Here's how the part is built. I have some questions about the finished solid (model axes, mm). A direction names the side the tool comes from. Coordinates: 2 decimals unless noted, no trailing zeros. Loops run counter-clockwise (first coordinate to the right, second up) from the corner with the lowest first, then second, coordinate; pieces in that order, holes last. Notation, with made-up numbers: (44.5, 52) -> (51.5, 52) arc R24 ccw to (51.5, 78) -> close; hole circle Ø2 at (82.25, -36). An arc over 180 degrees is marked (long way). Use CSV: the item, a comma, the result in double quotes. Start each with the question number.
from build123d import *

# Parameters (mm, degrees)
EXTRUDE_1_DEPTH = 2.2


with BuildPart() as part:
    # Model → 凸台-拉伸1 (new body)
    with BuildSketch(Plane.XY):
        Polygon((-11.407474747, -25.191111111), (-11.407474747, -22.191111111), (-16.407474747, -22.191111111), (-16.407474747, -19.191111111), (-21.407474747, -19.191111111), (-21.407474747, -14.191111111), (-23.407474747, -14.191111111), (-23.407474747, -4.191111111), (-21.407474747, -4.191111111), (-21.407474747, 5.808888889), (-23.407474747, 5.808888889), (-23.407474747, 15.808888889), (-21.407474747, 15.808888889), (-21.407474747, 20.808888889), (-16.407474747, 20.808888889), (-16.407474747, 23.808888889), (-11.407474747, 23.808888889), (-11.407474747, 26.808888889), (-1.407474747, 26.808888889), (-1.407474747, 23.808888889), (3.592525253, 23.808888889), (3.592525253, 26.808888889), (13.592525253, 26.808888889), (13.592525253, 23.808888889), (18.592525253, 23.808888889), (18.592525253, 20.808888889), (23.592525253, 20.808888889), (23.592525253, 15.808888889), (25.592525253, 15.808888889), (25.592525253, 5.808888889), (23.592525253, 5.808888889), (23.592525253, -4.191111111), (25.592525253, -4.191111111), (25.592525253, -14.191111111), (23.592525253, -14.191111111), (23.592525253, -19.191111111), (18.592525253, -19.191111111), (18.592525253, -22.191111111), (13.592525253, -22.191111111), (13.592525253, -25.191111111), (3.592525253, -25.191111111), (3.592525253, -22.191111111), (-1.407474747, -22.191111111), (-1.407474747, -25.191111111), align=None)
        with BuildLine():
            Line((16.092525253, 13.808888889), (15.092525253, 13.808888889))
            ThreePointArc((15.092525253, 13.808888889), (14.031865081, 14.248228717), (13.592525253, 15.308888889))
            Line((13.592525253, 15.308888889), (13.592525253, 16.308888889))
            ThreePointArc((13.592525253, 16.308888889), (13.153185424, 17.369549061), (12.092525253, 17.808888889))
            Line((12.092525253, 17.808888889), (-9.907474747, 17.808888889))
            ThreePointArc((-9.907474747, 17.808888889), (-10.968134919, 17.369549061), (-11.407474747, 16.308888889))
            Line((-11.407474747, 16.308888889), (-11.407474747, 15.308888889))
            ThreePointArc((-11.407474747, 15.308888889), (-11.846814576, 14.248228717), (-12.907474747, 13.808888889))
            Line((-12.907474747, 13.808888889), (-13.907474747, 13.808888889))
            ThreePointArc((-13.907474747, 13.808888889), (-14.968134919, 13.369549061), (-15.407474747, 12.308888889))
            Line((-15.407474747, 12.308888889), (-15.407474747, -10.691111111))
            ThreePointArc((-15.407474747, -10.691111111), (-14.968134919, -11.751771283), (-13.907474747, -12.191111111))
            Line((-13.907474747, -12.191111111), (-12.907474747, -12.191111111))
            ThreePointArc((-12.907474747, -12.191111111), (-11.846814576, -12.630450939), (-11.407474747, -13.691111111))
            Line((-11.407474747, -13.691111111), (-11.407474747, -14.691111111))
            ThreePointArc((-11.407474747, -14.691111111), (-10.968134919, -15.751771283), (-9.907474747, -16.191111111))
            Line((-9.907474747, -16.191111111), (12.092525253, -16.191111111))
            ThreePointArc((12.092525253, -16.191111111), (13.153185424, -15.751771283), (13.592525253, -14.691111111))
            Line((13.592525253, -14.691111111), (13.592525253, -13.691111111))
            ThreePointArc((13.592525253, -13.691111111), (14.031865081, -12.630450939), (15.092525253, -12.191111111))
            Line((15.092525253, -12.191111111), (16.092525253, -12.191111111))
            ThreePointArc((16.092525253, -12.191111111), (17.153185424, -11.751771283), (17.592525253, -10.691111111))
            Line((17.592525253, -10.691111111), (17.592525253, 12.308888889))
            ThreePointArc((17.592525253, 12.308888889), (17.153185424, 13.369549061), (16.092525253, 13.808888889))
        make_face(mode=Mode.SUBTRACT)
    extrude(amount=EXTRUDE_1_DEPTH)


solid = part.part
1) I want a section at B-B, the plane y = 14.5. Please give me the cut outline in (x, z).
2) I want a section at A-A, the plane x = -6.5. Please give me the cut outline in (y, z).
3) Please list where these lines run through material, in increasing order: L1, parallel to X at y = 11, z = 0.9; L2, parallel to Y at x = 2, z = 0.75; L3, parallel to X at y = 16.5, z = 0.6. Write a range as [from, to].
4) I want a section at D-D, the plane y = 22. Please give me the cut outline in (x, z), plus the area to 3 significant figures.
5) I want a section at C-C, the plane x = 20.5. Please give me the cut outline in (y, z), plus the area to 3 significant figures.
6) Thinking about a two-plate mould opening in X: for faces 1 (the face through (13.593, 25, 1)), 2 (the face through (-14.96, 13.38, 1.08)), 3 (the face through (16, -22.191, 1)), which applies, pulls with the +X half, pulls with the -X half, needs draft (parallel to the pull), parting line crosses it, or undercut?
7) For P1, Ø0.7, axis at y = 17.5, z = 1, coming from the -X side; P2, Ø0.7, axis at x = 0.5, z = 1, coming from the -Y side; P3, Ø0.6, axis at x = 24, z = 1, coming from the -Y side, each with a flat end and sliding along its axis, tell me the tip position at first contact or that it passes through.
8) Which directions (+Z, -Z, +X, -X, +Y, -Y) give clear straight access to the entire face, cutting with the end or side of a thin tool? Please do faces 4 (the face through (3.593, 25, 1)), 5 (the face through (-22, -4.191, 1)), 6 (the face through (17.1, -11.8, 1.1)), 7 (the face through (-11.407, 25, 1)), 8 (the face through (25, -14.191, 1)).
Return value:
1,outline,"(-23.41, 0) -> (-11.64, 0) -> (-11.64, 2.2) -> (-23.41, 2.2) -> close; (13.83, 0) -> (25.59, 0) -> (25.59, 2.2) -> (13.83, 2.2) -> close"
2,outline,"(-25.19, 0) -> (-16.19, 0) -> (-16.19, 2.2) -> (-25.19, 2.2) -> close; (17.81, 0) -> (26.81, 0) -> (26.81, 2.2) -> (17.81, 2.2) -> close"
3,L1,"x = [-23.41, -15.41], [17.59, 25.59]"
3,L2,"y = [-22.19, -16.19], [17.81, 23.81]"
3,L3,"x = [-21.41, -11.4], [13.58, 23.59]"
4,outline,"(-16.41, 0) -> (18.59, 0) -> (18.59, 2.2) -> (-16.41, 2.2) -> close"
4,area,"77.0 mm²"
5,outline,"(-19.19, 0) -> (20.81, 0) -> (20.81, 2.2) -> (-19.19, 2.2) -> close"
5,area,"88.0 mm²"
6,face 1,"pulls with the +X half"
6,face 2,"undercut"
6,face 3,"needs draft"
7,P1,"stops at x = -21.41"
7,P2,"stops at y = -22.19"
7,P3,"stops at y = -14.19"
8,face 4,"+Z, -Z, +Y"
8,face 5,"+Z, -Z, -X"
8,face 6,"+Z, -Z"
8,face 7,"+Z, -Z, -X, +Y"
8,face 8,"+Z, -Z, +X, -Y"
